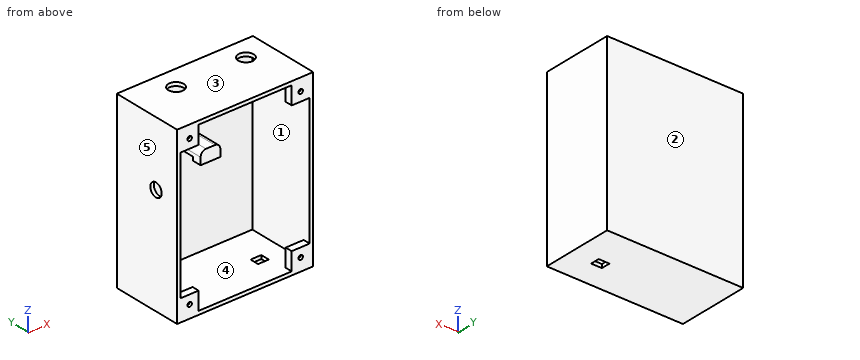
```python
from build123d import *

# Parameters (mm, degrees)
SKETCH1_W               = 76
SKETCH1_H               = 96
BOSS_EXTRUDE1_DEPTH     = 40
SKETCH2_W               = 72
SKETCH2_H               = 92
CUT_EXTRUDE3_DEPTH      = 38
CUT_EXTRUDE4_REACH      = 112.725
SKETCH7_R               = 4.25
SKETCH10_W              = 11
SKETCH10_H              = 5
BOSS_EXTRUDE2_DEPTH     = 15
FILLET2_R               = 3
CUT_EXTRUDE5_REACH      = 110.995
SKETCH11_W              = 6
SKETCH11_H              = 5
SKETCH12_W              = 11
SKETCH12_H              = 5
BOSS_EXTRUDE3_DEPTH     = 2
CUT_EXTRUDE6_REACH      = 100.387
SKETCH13_R              = 3.75
SKETCH15_W              = 10
SKETCH15_H              = 10
SKETCH15_R              = 1.25
BOSS_EXTRUDE4_DEPTH     = 4
MIRROR2_COPY_1_SKETCH_W = 10
MIRROR2_COPY_1_SKETCH_H = 10
MIRROR2_COPY_1_SKETCH_R = 1.25
MIRROR2_COPY_1_DEPTH    = 4
SKETCH17_W              = 6
SKETCH17_H              = 6
CUT_EXTRUDE7_DEPTH      = 2.5
MIRROR4_COPY_1_SKETCH_W = 6
MIRROR4_COPY_1_SKETCH_H = 6
MIRROR4_COPY_1_DEPTH    = 2.5


with BuildPart() as part:
    # Sketch1 → Boss-Extrude1 (new body)
    with BuildSketch(Plane(origin=(0, 0, 0), x_dir=(1, 0, 0), z_dir=(0, 1, 0))):
        Rectangle(SKETCH1_W, SKETCH1_H)
    extrude(amount=BOSS_EXTRUDE1_DEPTH)

    # Sketch2 → Cut-Extrude3 (cut)
    with BuildSketch(Plane.XZ):
        Rectangle(SKETCH2_W, SKETCH2_H)
    extrude(amount=-CUT_EXTRUDE3_DEPTH, mode=Mode.SUBTRACT)

    # Sketch7 → Cut-Extrude4 (cut, up to next)
    with BuildSketch(Plane.XY.offset(48), mode=Mode.PRIVATE) as cut_extrude4_sk1:
        with Locations((-15, 28)):
            Circle(SKETCH7_R)
    cut_extrude4_tool1 = extrude(cut_extrude4_sk1.sketch, amount=-CUT_EXTRUDE4_REACH, mode=Mode.PRIVATE) & part.part
    # Sketch7 → Cut-Extrude4 (cut, up to next)
    with BuildSketch(Plane.XY.offset(48), mode=Mode.PRIVATE) as cut_extrude4_sk2:
        with Locations((24, 28)):
            Circle(SKETCH7_R)
    cut_extrude4_tool2 = extrude(cut_extrude4_sk2.sketch, amount=-CUT_EXTRUDE4_REACH, mode=Mode.PRIVATE) & part.part
    add(cut_extrude4_tool1.solids().sort_by_distance((-15, 28, 48))[0], mode=Mode.SUBTRACT)
    add(cut_extrude4_tool2.solids().sort_by_distance((24, 28, 48))[0], mode=Mode.SUBTRACT)

    # Sketch10 → Boss-Extrude2 (add)
    with BuildSketch(Plane.XZ.offset(-38)):
        with Locations((0, 12.5)):
            Rectangle(SKETCH10_W, SKETCH10_H)
    extrude(amount=BOSS_EXTRUDE2_DEPTH)

    # Fillet2
    fillet2_edges = [part.edges().sort_by_distance(p)[0] for p in [
        (5.5, 30.5, 15),
        (-5.5, 30.5, 15),
    ]]
    fillet(fillet2_edges, radius=FILLET2_R)

    # Sketch11 → Cut-Extrude5 (cut, up to next)
    with BuildSketch(Plane.XY.offset(-46), mode=Mode.PRIVATE) as cut_extrude5_sk1:
        with Locations((22, 16.5)):
            Rectangle(SKETCH11_W, SKETCH11_H)
    cut_extrude5_tool1 = extrude(cut_extrude5_sk1.sketch, amount=-CUT_EXTRUDE5_REACH, mode=Mode.PRIVATE) & part.part
    add(cut_extrude5_tool1.solids().sort_by_distance((22, 16.5, -46))[0], mode=Mode.SUBTRACT)

    # Sketch12 → Boss-Extrude3 (add)
    with BuildSketch(Plane(origin=(0, 0, 10), x_dir=(-1, 0, 0), z_dir=(0, 0, -1))):
        with Locations((0, 25.5)):
            Rectangle(SKETCH12_W, SKETCH12_H)
    extrude(amount=BOSS_EXTRUDE3_DEPTH)

    # Sketch13 → Cut-Extrude6 (cut, up to next)
    with BuildSketch(Plane.ZY.offset(38), mode=Mode.PRIVATE) as cut_extrude6_sk1:
        with Locations((12, 14)):
            Circle(SKETCH13_R)
    cut_extrude6_tool1 = extrude(cut_extrude6_sk1.sketch, amount=-CUT_EXTRUDE6_REACH, mode=Mode.PRIVATE) & part.part
    add(cut_extrude6_tool1.solids().sort_by_distance((-38, 14, 12))[0], mode=Mode.SUBTRACT)

    # Sketch15 → Boss-Extrude4 (add)
    with BuildSketch(Plane.XZ):
        with Locations((31, 41)):
            Rectangle(SKETCH15_W, SKETCH15_H)
        with Locations(Location((31, 41, 0), (0, 0, 270))):
            Circle(SKETCH15_R, mode=Mode.SUBTRACT)
    boss_extrude4 = extrude(amount=-BOSS_EXTRUDE4_DEPTH)

    # Mirror1: Boss-Extrude4 across plane
    add(boss_extrude4.mirror(Plane(origin=(0, 0, 0), x_dir=(0, 0, 1), z_dir=(1, 0, 0))))

    # Mirror2: Boss-Extrude4 across plane
    add(boss_extrude4.mirror(Plane.XY))

    # Mirror2 copy 1 sketch → Mirror2 copy 1 (add)
    with BuildSketch(Plane(origin=(0, 0, 0), x_dir=(-1, 0, 0), z_dir=(0, -1, 0))):
        with Locations((31, 41)):
            Rectangle(MIRROR2_COPY_1_SKETCH_W, MIRROR2_COPY_1_SKETCH_H)
        with Locations(Location((31, 41, 0), (0, 0, 270))):
            Circle(MIRROR2_COPY_1_SKETCH_R, mode=Mode.SUBTRACT)
    extrude(amount=-MIRROR2_COPY_1_DEPTH)

    # Sketch17 → Cut-Extrude7 (cut)
    with BuildSketch(Plane(origin=(0, 4, 0), x_dir=(1, 0, 0), z_dir=(0, 1, 0))):
        with Locations((31, -41)):
            Rectangle(SKETCH17_W, SKETCH17_H)
    cut_extrude7 = extrude(amount=-CUT_EXTRUDE7_DEPTH, mode=Mode.SUBTRACT)

    # Mirror3: Cut-Extrude7 across plane
    add(cut_extrude7.mirror(Plane(origin=(0, 0, 0), x_dir=(0, 0, 1), z_dir=(1, 0, 0))), mode=Mode.SUBTRACT)

    # Mirror4: Cut-Extrude7 across plane
    add(cut_extrude7.mirror(Plane.XY), mode=Mode.SUBTRACT)

    # Mirror4 copy 1 sketch → Mirror4 copy 1 (cut)
    with BuildSketch(Plane(origin=(0, 4, 0), x_dir=(-1, 0, 0), z_dir=(0, 1, 0))):
        with Locations((31, -41)):
            Rectangle(MIRROR4_COPY_1_SKETCH_W, MIRROR4_COPY_1_SKETCH_H)
    extrude(amount=-MIRROR4_COPY_1_DEPTH, mode=Mode.SUBTRACT)


solid = part.part
```
CAD build for the part. Positions are in the model's coordinates, mm. Face numbers are marked on the shaded views. A direction names the side the tool comes from. Coordinates: 2 decimals unless noted, no trailing zeros. Order: outer loops, then holes, each group sorted by start corner. A loop starts at its lowest first (then second) coordinate and runs counter-clockwise, first axis right, second up. Notation, with made-up numbers: (0, 66.5) - (33, 66.5) arc R28 cw to (33, 90.5) - close; hole circle Ø3 at (37.5, 77). An arc over 180 degrees is marked (long way). Answer in a Markdown table with one row per item.
1. Slice it at A-A, the plane y = 8. List the corners of the cut face in (x, z).
Answer:
| item | result |
|---|---|
| outline | (-38, -48) - (38, -48) - (38, 48) - (-38, 48) - close; hole (-36, -46) - (36, -46) - (36, 46) - (-36, 46) - close |
2. Pull direction X, two halves, no side cores. Call the marked faces 3, 4 and 5: +X half, -X half, draft (parallel to the pull), parting line (faces both ways), or undercut.
Answer:
| item | result |
|---|---|
| face 3 | draft |
| face 4 | undercut |
| face 5 | -X half |
3. Slice it at D-D, the plane x = -31. List the corners of the cut face in (y, z).
Answer:
| item | result |
|---|---|
| outline | (0, -48) - (40, -48) - (40, 48) - (0, 48) - (0, 42.25) - (1.5, 42.25) - (1.5, 44) - (4, 44) - (4, 46) - (38, 46) - (38, -46) - (4, -46) - (4, -44) - (1.5, -44) - (1.5, -42.25) - (0, -42.25) - close; (0, -39.75) - (1.5, -39.75) - (1.5, -38) - (4, -38) - (4, -36) - (0, -36) - close; (0, 36) - (4, 36) - (4, 38) - (1.5, 38) - (1.5, 39.75) - (0, 39.75) - close |
4. Slice it at B-B, the plane x = -15. List the corners of the cut face in (y, z), then the cut area to 3 significant figures.
Answer:
| item | result |
|---|---|
| outline | (0, -48) - (40, -48) - (40, 48) - (32.25, 48) - (32.25, 46) - (38, 46) - (38, -46) - (0, -46) - close; (0, 46) - (23.75, 46) - (23.75, 48) - (0, 48) - close |
| area | 327 mm² |
5. Drill centre lines: L1, parallel to X at y = 25.5, z = 9; L2, parallel to X at y = 0.8, z = 41; L3, parallel to Z at x = -31, y = 0.35. Where is each one in solid material? Low to high. Write a range as from..to.
Answer:
| item | result |
|---|---|
| L1 | -38..-36, -5.5..5.5, 36..38 |
| L2 | -38..-32.25, -29.75..-26, 26..29.75, 32.25..38 |
| L3 | -48..-42.25, -39.75..-36, 36..39.75, 42.25..48 |
6. Slice it at C-C, the plane z = -41. List the corners of the cut face in (x, y), then the cut area to 4 significant figures.
Answer:
| item | result |
|---|---|
| outline | (-38, 0) - (-32.25, 0) - (-32.25, 1.5) - (-34, 1.5) - (-34, 4) - (-36, 4) - (-36, 38) - (36, 38) - (36, 4) - (34, 4) - (34, 1.5) - (32.25, 1.5) - (32.25, 0) - (38, 0) - (38, 40) - (-38, 40) - close; (-29.75, 0) - (-26, 0) - (-26, 4) - (-28, 4) - (-28, 1.5) - (-29.75, 1.5) - close; (26, 0) - (29.75, 0) - (29.75, 1.5) - (28, 1.5) - (28, 4) - (26, 4) - close |
| area | 346.5 mm² |
7. Flat gauge pins, fed straight in: P1, Ø5, axis at x = -15, y = 28, coming from the +Z side; P2, Ø7.5, axis at x = -0.5, z = 12, coming from the -Y side; P3, Ø8, axis at x = 15, z = 15, coming from the -Y side. Where does each tip first touch, or does it go through?
Answer:
| item | result |
|---|---|
| P1 | z = -46 |
| P2 | y = 23 |
| P3 | y = 38 |
8. 3-axis set-ups, long thin cutter, end or side, ignore diameter. For the marked faces 1 and 2: which of +Z, -Z, +X, -X, +Y, -Y reach the whole face in a straight line?
Answer:
| item | result |
|---|---|
| face 1 | none |
| face 2 | +Z, -Z, +X, -X, +Y |
